Autodesk Inventor part; units mm, degrees
ref_plane "YZ Plane" through (0, 0, 0) normal (1, 0, 0) x (0, 1, 0)
ref_plane "XZ Plane" through (0, 0, 0) normal (0, 1, 0) x (-1, 0, 0)
ref_plane "XY Plane" through (0, 0, 0) normal (0, 0, 1) x (1, 0, 0)
sketch "Sketch1" plane through (0, 0, 0) normal (0, 0, 1) x (1, 0, 0)
  line L0 (0, 0) -> (47, 0)
  line L1 (47, 0) -> (47, -300)
  line L2 (47, -300) -> (0, -300)
  line L3 (0, -300) -> (0, 0)
  dimension "d0" = 47
  dimension "d1" = 300
extrude "Extrusion1" add sketch "Sketch1" along normal blind 25.4
sketch "Sketch2" plane through (0, -300, 0) normal (0, -1, 0) x (1, 0, 0)
  line L0 (0, 0) -> (0, 25.4)
  line L1 (0, 25.4) -> (47, 25.4)
  line L2 (0, 0) -> (10, 0)
  line L3 (10, 0) -> (10, 21.4)
  line L4 (10, 25.4) -> (0, 25.4)
  line L5 (0, 25.4) -> (0, 0)
  line L6 (0, 0) -> (47, 0)
  line L7 (47, 0) -> (37, 0)
  line L8 (37, 0) -> (37, 25.4)
  line L9 (37, 25.4) -> (47, 25.4)
  line L10 (47, 25.4) -> (47, 0)
  line L11 (10, 25.4) -> (3.1941, 0)
  line L12 (10, 25.4) -> (36.296, 25.4) construction
  line L13 (37, 25.4) -> (43.8059, 0)
  line L14 (37, 25.4) -> (63.296, 25.4) construction
  line L15 (37, 25.4) -> (37, 21.4)
  line L16 (37, 21.4) -> (8.9282, 21.4)
  line L17 (37, 21.4) -> (38.0718, 21.4)
  line L18 (10, 25.4) -> (37, 25.4)
  dimension "d4" = 10
  dimension "d5" = 10
  dimension "d6" = 105
  dimension "d7" = 75
  dimension "d8" = 4
extrude "Extrusion2" cut sketch "Sketch2" against normal blind 300 contours L1 L8 L16 L11 | L13 L17 L8
sketch "Sketch3" plane through (0, 0, 0) normal (0, 0, -1) x (-1, 0, 0)
  line L0 (-50.8, -30) -> (0, -30)
  line L1 (0, -30) -> (-50.8, -30)
  line L2 (0, 8.1) -> (0, -30)
  line L3 (-47, -30) -> (0, -30)
  line L4 (0, -15) -> (0, -30)
  line L5 (0, -30) -> (-47, -30)
  line L6 (-47, -30) -> (-47, -15)
  line L7 (-47, -15) -> (0, -15)
  line L8 (0, -15) -> (-47, -30) construction
  line L9 (0, -30) -> (-47, -15) construction
  line L10 (-47, 0) -> (0, 0)
  line L11 (0, 0) -> (-47, -15) construction
  line L12 (0, -15) -> (-47, 0) construction
  line L13 (-47, -15) -> (0, -15)
  line L14 (0, -15) -> (-47, -15)
  line L15 (0, 0) -> (0, -15)
  line L16 (-47, -15) -> (-47, 0)
  line L17 (-8.5, -22.5) -> (-8.5, -7.5)
  circle A0 centre (-8.5, -22.5) radius 1.5875
  circle A1 centre (-38.5, -22.5) radius 1.5875
  circle A2 centre (-38.5, -7.5) radius 1.5875
  circle A3 centre (-8.5, -7.5) radius 1.5875
  line L18 (-47, 0) -> (0, 0)
  line L19 (0, 0) -> (0, -122.988)
  line L20 (0, 0) -> (0, -300)
  line L21 (-50.8, -122.988) -> (0, -122.988)
  line L22 (0, -122.988) -> (-50.8, -122.988)
  line L23 (-47, -122.988) -> (0, -122.988)
  line L24 (0, -107.988) -> (0, -122.988)
  line L25 (0, -122.988) -> (-47, -122.988)
  line L26 (-47, -122.988) -> (-47, -107.988)
  line L27 (-47, -107.988) -> (0, -107.988)
  line L28 (0, -107.988) -> (-47, -122.988) construction
  line L29 (0, -122.988) -> (-47, -107.988) construction
  line L30 (-47, -92.988) -> (0, -92.988)
  line L31 (0, -92.988) -> (-47, -107.988) construction
  line L32 (0, -107.988) -> (-47, -92.988) construction
  line L33 (-47, -107.988) -> (0, -107.988)
  line L34 (0, -107.988) -> (-47, -107.988)
  line L35 (0, -92.988) -> (0, -107.988)
  line L36 (-47, -107.988) -> (-47, -92.988)
  line L37 (-8.5, -115.488) -> (-8.5, -100.488)
  circle A4 centre (-8.5, -115.488) radius 1.5875
  circle A5 centre (-38.5, -115.488) radius 1.5875
  circle A6 centre (-38.5, -100.488) radius 1.5875
  circle A7 centre (-8.5, -100.488) radius 1.5875
  line L38 (-16, -115.488) -> (-13.5, -115.488)
  line L39 (-13.5, -115.488) -> (-8.5, -115.488)
  line L40 (-31, -115.488) -> (-33.5, -115.488)
  line L41 (-33.5, -115.488) -> (-41, -115.488)
  line L42 (-41, -115.488) -> (-38.5, -115.488)
  point P0 (0, -6.35)
  point P1 (0, -30)
  point P2 (-27, -15)
  point P3 (-12, -15)
  point P4 (0, -15)
  point P5 (-10, 0)
  point P6 (0, -99.338)
  point P7 (-27, -107.988)
  point P8 (-12, -107.988)
  point P9 (0, -107.988)
  dimension "d11" = 15
  dimension "d12" = 15
  dimension "d13" = 3.175
  dimension "d14" = 3.175
  dimension "d15" = 3.175
  dimension "d16" = 3.175
  dimension "d17" = 122.988
  dimension "d18" = 15
  dimension "d19" = 15
  dimension "d20" = 3.175
  dimension "d21" = 3.175
  dimension "d22" = 3.175
  dimension "d23" = 3.175
  dimension "d30" = 5
  dimension "d31" = 7.5
  dimension "d32" = 2.5
extrude "Extrusion3" cut sketch "Sketch3" against normal blind 10 contours A0 | A7 | A3 | A4 L39 L37 | L37 L39 A4 | A1 | A2 | L41 A5 | A5 L41 | A6
sketch "Sketch4" plane through (0, -300, 0) normal (0, -1, 0) x (1, 0, 0)
  line L0 (0, 0) -> (47, 0)
  line L1 (47, 0) -> (47, 25.4)
  line L2 (0, 0) -> (47, 0)
  line L3 (47, 0) -> (47, 12.7)
  line L4 (47, 12.7) -> (0, 12.7)
  line L5 (0, 12.7) -> (0, 0)
  dimension "d27" = 12.7
extrude "Extrusion4" cut sketch "Sketch4" against normal blind 160
sketch "Sketch7" plane through (0, 0, 0) normal (0, 1, 0) x (1, 0, 0)
  line L0 (47, -25.4) -> (37, -25.4)
  line L1 (0, 0) -> (47, -25.4)
  line L2 (47, -25.4) -> (47, 0)
  line L3 (10, -25.4) -> (0, -25.4)
  line L4 (47, 0) -> (0, -25.4)
  circle A0 centre (23.5, -12.7) radius 6.35
  line L5 (23.5, -12.7) -> (21, -12.7)
  line L6 (0, -12.7) -> (47, -12.7)
  line L7 (23.5, -12.7) -> (23.5, -10.2)
  line L8 (23.5, -12.7) -> (26, -12.7) construction
  circle A1 centre (23.5, -10.2) radius 6.35
  dimension "d33" = 12.7
  dimension "d34" = 2.5
  dimension "d35" = 2.5
  dimension "d36" = 90
  dimension "d37" = 12.7
extrude "Extrusion5" cut sketch "Sketch7" against normal blind 100 contours A1 L4 A0 L1 | L1 A0 A1 | A0 L4 L1 | L1 L5 L6 A1 A0 | A1 A0 L4 | L6 A1 L1 | L1 A1 L4 | L4 A1 L6 L5 | L4 A0 A1 L6 picked at (23.5, -5.5468) picked at (27.3983, -11.8828)
sketch "Sketch9" plane through (0, 0, 0) normal (0, 0, -1) x (-1, 0, 0)
  circle A0 centre (-38.5, -22.5) radius 1.5875
  circle A1 centre (-38.5, -100.488) radius 1.5875
  line L0 (-38.5, -22.5) -> (-38.5, -100.488)
  line L1 (-38.5, -100.488) -> (-38.5, -62.7)
  circle A2 centre (-38.5, -115.488) radius 1.5875
  line L2 (-38.5, -115.488) -> (-38.5, -77.7)
  circle A3 centre (-38.5, -62.7) radius 1.5875
  circle A4 centre (-38.5, -77.7) radius 1.5875
  line L3 (-38.5, -100.488) -> (-8.5476, -100.488)
  line L4 (-38.5, -77.7) -> (-8.4125, -77.7)
  circle A5 centre (-8.4125, -62.7) radius 1.5875
  circle A6 centre (-8.4125, -77.7) radius 1.5875
  line L5 (-10, -62.7) -> (-11.5875, -62.7)
  point P0 (0, 0)
  dimension "d40" = 37.788
  dimension "d41" = 37.788
  dimension "d42" = 3.175
  dimension "d43" = 3.175
  dimension "d44" = 3.175
  dimension "d45" = 3.175
  dimension "d59" = 1.5875
extrude "Extrusion6" cut sketch "Sketch9" against normal blind 10 contours A6 | A4 L4 L0 | L0 A4 | A3 L0 | L0 A3 | L4 A4 L0 | A5
sketch "Sketch10" plane through (0, 0, 0) normal (0, 0, -1) x (-1, 0, 0)
  line L0 (-47, -140) -> (-47, 0)
  line L1 (0, 0) -> (-47, 0)
  line L2 (-47, 0) -> (-47, -50)
  line L3 (-47, -50) -> (0, -50)
  line L4 (0, -50) -> (0, 0)
  point P0 (-47, 0)
  dimension "d48" = 50
extrude "Extrusion7" cut sketch "Sketch10" against normal blind 30
sketch "Sketch11" plane through (0, 0, 0) normal (0, 0, -1) x (-1, 0, 0)
  line L0 (-10, -50) -> (0, -50)
  line L1 (0, -50) -> (1.9, -50)
  line L2 (0, -50) -> (-47, -50)
  line L3 (-47, -50) -> (-48.9, -50)
  line L4 (-48.9, -50) -> (-48.9, -300)
  line L5 (-37, -300) -> (-47, -300)
  line L6 (-47, -300) -> (-48.9, -300)
  line L7 (-47, -300) -> (-47, -50)
  line L8 (-47, -50) -> (-47, -300)
  line L9 (0, -50) -> (0, -300)
  line L10 (0, -50) -> (0, -300)
  line L11 (0, -300) -> (0, -298.1)
  line L12 (1.9, -300) -> (0, -300)
  line L13 (1.9, -300) -> (1.9, -50)
  point P0 (0, 0)
  dimension "d51" = 1.9
  dimension "d52" = 1.9
  dimension "d53" = 1.9
extrude "Extrusion8" add sketch "Sketch11" against normal blind 25.4
sketch "Sketch12" plane through (0, 0, 0) normal (0, 0, -1) x (-1, 0, 0)
  line L0 (-37, -300) -> (-48.9, -300)
  line L1 (1.9, -50) -> (1.9, -300)
  line L2 (-48.9, -300) -> (1.9, -300)
  line L3 (1.9, -300) -> (1.9, -140)
  line L4 (1.9, -140) -> (-48.9, -140)
  line L5 (-48.9, -140) -> (-48.9, -300)
  point P0 (0, 0)
  dimension "d56" = 160
extrude "Extrusion9" cut sketch "Sketch12" against normal blind 12.7
properties part number "5211_Bias_TxRx_Relative_Dovetail_Female_MPSv2_v4" material "Polyethylene, High Density"
Here's how the part is built. I have some questions about the finished solid (model axes, mm). A direction names the side the tool comes from. Round coordinates to 2 decimals unless told otherwise and drop trailing zeros. Order: outer loops, then holes, each group sorted by start corner. A loop starts at its lowest first (then second) coordinate and runs counter-clockwise, first axis right, second up. Notation, with made-up numbers: (-11.75, 79) -> (-5.75, 79) arc R16 cw to (-5.75, 85) -> close; hole circle Ø4 at (-5, 81.25). An arc over 180 degrees is marked (long way). Use CSV: the item, a comma, the result in double quotes.
1. I want a section at B-B on z = 7.25. Give the number of separate pieces and of enclosed holes in the cut face, and give its area (3 significant figures).
Recorded:
separate pieces,"1"
enclosed holes,"8"
area,"3,950 mm2"
2. I want a section at D-D on x = 3.5. List the corners of the cut face in (y, z) for me.
Recorded:
outline,"(-300, 12.7) -> (-140, 12.7) -> (-140, 0) -> (-50, 0) -> (-50, 25.4) -> (-300, 25.4) -> close"
3. Thinking about a two-plate mould opening in Z: for faces 5 (the face through (9.472, -176.75, 23.428)), 6 (the face through (48.9, -145, 15)), 7 (the face through (24, -219, 12.7)), which applies, pulls with the +Z half, pulls with the -Z half, needs draft (parallel to the pull), parting line crosses it, or undercut?
Recorded:
face 5,"undercut"
face 6,"needs draft"
face 7,"pulls with the -Z half"
4. Which directions (+Z, -Z, +X, -X, +Y, -Y) give clear straight access to the entire face, cutting with the end or side of a thin tool? Please do faces 1 (the face through (37.528, -176.75, 23.428)), 2 (the face through (23, -100, 10)), 3 (the face through (4, -173, 25.4)), 4 (the face through (23, -140, 6)).
Recorded:
face 1,"+Y, -Y"
face 2,"+Y"
face 3,"+Z, +X, -X, +Y, -Y"
face 4,"-Z, +X, -X, -Y"
5. I want a section at C-C on x = 33.5. List the corners of the cut face in (y, z) for me, and give its area (3 significant figures).
Recorded:
outline,"(-300, 12.7) -> (-140, 12.7) -> (-140, 0) -> (-50, 0) -> (-50, 21.4) -> (-300, 21.4) -> close"
area,"3,320 mm2"
6. I need wall thicknesses on line 1 along Y through (x, z) = (38.5, 7.5); line 2 along X through (y, z) = (-61.5, 10.2); line 3 along Z through (x, y) = (35.5, -258). Which ranges of each line are inside material? Lowest first, please.
Recorded:
line 1,"y = -140 to -117.08, -113.9 to -102.08, -98.9 to -79.29, -76.11 to -64.29, -61.11 to -50"
line 2,"x = -1.9 to 17.15, 29.85 to 48.9"
line 3,"z = 12.7 to 21.4"
7. I'm going to push flat-ended pins straight in: P1, Ø6, axis at x = 14, z = 9.5, coming from the -Y side; P2, Ø1, axis at x = 8, y = -62.5, coming from the -Z side. Where does each tip first touch, or does it pass through?
Recorded:
P1,"stops at y = -140"
P2,"stops at z = 10"
8. I want a section at A-A on y = -276. List the corners of the cut face in (x, z) for me, and give its area (3 significant figures).
Recorded:
outline,"(-1.9, 12.7) -> (48.9, 12.7) -> (48.9, 25.4) -> (37, 25.4) -> (38.07, 21.4) -> (8.93, 21.4) -> (10, 25.4) -> (-1.9, 25.4) -> close"
area,"533 mm2"
